For this review, take the finished solid that the model builds, in its own axes (mm). A direction names the side the tool comes from. Coordinates: 2 decimals unless noted, no trailing zeros. Write each loop counter-clockwise with the first axis right and the second up, starting at its lowest first coordinate (ties: lowest second). Pieces come first, ordered by that corner, then holes.
1) We need section A-A on z = 1.5. Write out the cut boundary in (x, y), then the cut area to 3 significant figures.
2) Insertion check: P1, Ø4.5, axis at x = 94.87, z = 2.11, coming from the +Y side; P2, Ø6, axis at x = -18.5, z = 3.5, coming from the -Y side; P3, Ø1, axis at y = 8, z = 5.5, coming from the +X side. Each pin has a flat end and moves straight along its axis. Give the tip position at first contact, or say it passes through.
3) For faces 1 (the face through (-14, 5, 6)), 2 (the face through (21.573, 7, 2)), 3 (the face through (39, 4, 17.114)), list the 3-axis set-ups (+Z, -Z, +X, -X, +Y, -Y) from which the entire face can be reached by the end or side of a thin tool; tool diameter is ignored.
4) Mouldability with a two-part tool opening along Z and no side actions: class faces 4 (the face through (39, 4, -12.886)), 5 (the face through (93.16, 2.46, 1.73)), 6 (the face through (104.869, 2, 2)) as pulls with the +Z half, pulls with the -Z half, needs draft (parallel to the pull), parting line crosses it, or undercut.
5) We need section C-C on y = 7. Write out the cut boundary in (x, z).
6) To check wall thickness, follow line 1 along X through (y, z) = (9.25, 2.5); line 2 along X through (y, z) = (5.25, -9); line 3 along X through (y, z) = (1.5, 4.25). State the ranges of each line that lie inside material, in increasing order.
7) We need section B-B on z = -9.75. Write out the cut boundary in (x, y).
8) We need section D-D on x = 85. Write out the cut boundary in (y, z).
from build123d import *

# Parameters (mm, degrees)
SKETCH_1_W          = 129
SKETCH_1_H          = 30
SKETCH_1_R          = 2.75
SKETCH_1_R_2        = 1.75
EXTRUDE_1_DEPTH     = 10
SKETCH_2_W          = 20
SKETCH_2_H          = 5
SKETCH_2_W_2        = 83.295582585
CUT_EXTRUDE_1_DEPTH = 110.532870251


with BuildPart() as part:
    # 草图1 → 凸台-拉伸1 (new body)
    with BuildSketch(Plane(origin=(0, 0, 0), x_dir=(1, 0, 0), z_dir=(0, 1, 0))):
        with Locations((40.368725869, -2.113899614)):
            Rectangle(SKETCH_1_W, SKETCH_1_H)
        with Locations(Location((-14.131274131, -2.113899614, 0), (0, 0, 270))):
            Circle(SKETCH_1_R, mode=Mode.SUBTRACT)
        with Locations(Location((94.868725869, -2.113899614, 0), (0, 0, 270))):
            Circle(SKETCH_1_R_2, mode=Mode.SUBTRACT)
    extrude(amount=EXTRUDE_1_DEPTH)

    # 草图2 → 切除-拉伸1 (cut, through all)
    with BuildSketch(Plane.XY.offset(17.113899614)):
        with Locations((-14.131274131, 2.5)):
            Rectangle(SKETCH_2_W, SKETCH_2_H)
        with Locations((63.220934576, 7.5)):
            Rectangle(SKETCH_2_W_2, SKETCH_2_H)
    extrude(amount=-CUT_EXTRUDE_1_DEPTH, mode=Mode.SUBTRACT)


solid = part.part
Result:
1. outline: (-24.13, 5) - (-16.81, 5) - (-16.81, 10) - (-24.13, 10) - close; (-11.45, 5) - (-4.13, 5) - (-4.13, 0) - (93.23, 0) - (93.23, 5) - (21.57, 5) - (21.57, 10) - (-11.45, 10) - close; (96.51, 0) - (104.87, 0) - (104.87, 5) - (96.51, 5) - close
1. area: 730 mm2
2. P1: stops at y = 5
2. P2: stops at y = 5
2. P3: stops at x = 21.57
3. face 1: +Z, -Z, -X, -Y
3. face 2: +Z, -Z, +X, +Y
3. face 3: +Z, +X, -X, +Y, -Y
4. face 4: pulls with the -Z half
4. face 5: undercut
4. face 6: needs draft
5. outline: (-24.13, -12.89) - (21.57, -12.89) - (21.57, 17.11) - (-24.13, 17.11) - close; hole circle Ø5.5 at (-14.13, 2.11)
6. line 1: x = -24.13 to -16.85, -11.41 to 21.57
6. line 2: x = -24.13 to 21.57
6. line 3: x = -4.13 to 104.87
7. outline: (-24.13, 5) - (-4.13, 5) - (-4.13, 0) - (104.87, 0) - (104.87, 5) - (21.57, 5) - (21.57, 10) - (-24.13, 10) - close
8. outline: (0, -12.89) - (5, -12.89) - (5, 17.11) - (0, 17.11) - close
